For this review, take the finished solid that the model builds, in its own axes (mm). A direction names the side the tool comes from. Give positions to 0.01 mm unless a question says otherwise; leave off trailing zeros. Order: outer loops, then holes, each group sorted by start corner. A loop starts at its lowest first (then second) coordinate and runs counter-clockwise, first axis right, second up. Notation, with made-up numbers: (-3, 74.25) - (34, 74.25) arc R21 ccw to (34, 113.25) - close; hole circle Ø8 at (-18.75, 22). An arc over 180 degrees is marked (long way). Answer as a JSON object with one key per item and string values. Group by question number.
from build123d import *

# Parameters (mm, degrees)
F0_R     = 6.35
F1_DEPTH = 2.54
F2_R     = 3.175
F3_DEPTH = 5.08
F4_R     = 3.175
F4_W     = 17.78
F4_H     = 12.7
F5_DEPTH = 5.08
F7_R     = 5.07999
F8_R     = 3.175
F9_DEPTH = 5.08


# Not quite as in the source:
# - a fillet or chamfer is up to 0.001 mm smaller than in the source, because OpenCascade refuses the exact size


with BuildPart() as f1:
    # F0 (on Front) → F1 (new body)
    with BuildSketch(Plane.XZ):
        with Locations((0, 22.225)):
            Circle(F0_R)
    extrude(amount=F1_DEPTH)

    # F2 (on face) → F3 (join)
    with BuildSketch(Plane.XZ.offset(2.54)):
        with Locations((0, 22.225)):
            Circle(F2_R)
    extrude(amount=F3_DEPTH)

    # F4 (on face) → F5 (join)
    with BuildSketch(Plane.XZ.offset(7.62)):
        with BuildLine():
            ThreePointArc((4.9490759915, 23.3708825552), (5.0471628682, 22.8016688665), (5.08, 22.225))
            ThreePointArc((5.08, 22.225), (-0.5766688665, 17.1778371318), (-4.9490759915, 23.3708825552))
            Line((-4.9490759915, 23.3708825552), (-8.89, 6.35))
            Line((-8.89, 6.35), (8.89, 6.35))
            Line((8.89, 6.35), (4.9490759915, 23.3708825552))
        make_face()
        with BuildLine():
            ThreePointArc((-4.9490759915, 23.3708825552), (-0.5766688665, 17.1778371318), (5.08, 22.225))
            ThreePointArc((5.08, 22.225), (5.0471628682, 22.8016688665), (4.9490759915, 23.3708825552))
            ThreePointArc((4.9490759915, 23.3708825552), (0, 27.305), (-4.9490759915, 23.3708825552))
        make_face()
        with Locations((0, 22.225)):
            Circle(F4_R, mode=Mode.SUBTRACT)
        with Locations((0, 22.225)):
            Circle(F4_R)
        Rectangle(F4_W, F4_H)
    extrude(amount=F5_DEPTH)

    # F6: F1 across plane


with BuildPart() as f1_1:
    add(f1.part)
    add(f1.part.mirror(Plane.XY))

    # F7 (radius 5.08 in the source; OpenCascade refuses exactly that, so slightly less here)
    f7_edges = [f1_1.edges().sort_by_distance(p)[0] for p in [
        (-8.89, -12.7, 0),
        (8.89, -12.7, 0),
    ]]
    fillet(f7_edges, radius=F7_R)

    # F8 (on face) → F9 (join)
    with BuildSketch(Plane.XZ.offset(12.7)):
        Circle(F8_R)
    extrude(amount=F9_DEPTH)


solid = f1_1.part
1) Consider section B-B (x = 0). Give the boundary of the cut face in (y, z) (3 decimals), plus the area to 3 significant figures.
2) Consider section C-C (x = 5.5). Give the boundary of the cut face in (y, z).
3) For pin 1 (3 mm diameter, centred on y = -11.5, z = -0.5, fed in from -X); pin 2 (5 mm diameter, centred on x = 2.5, y = -6.5, fed in from +Z); pin 3 (10 mm diameter, centred on x = 1, z = 21, fed in from -Y), all flat-tipped, find the tip position at first contact; note any pin that passes through.
4) For line 1 (Y direction, x = -3, z = -21); line 2 (Y direction, x = -5, z = 20); line 3 (Y direction, x = 2.5, z = 8.5), list the stretches that pass through material, from the lowest coordinate up.
5) Mouldability with a two-part tool opening along Y and no side actions: class faces 1 (the face through (6.51, -9.51, -16.63)), 2 (the face through (0, -17.78, 0)), 3 (the face through (-3, -2.54, 24)) as released by +Y, released by -Y, zero draft, split by the parting line, or undercut.
6) Consider section A-A (z = -18). Give the boundary of the cut face in (x, y).
7) For faces 4 (the face through (-6.454, -9.511, -16.871)), 5 (the face through (0.096, -10.124, -27.304)), 6 (the face through (-1.377, -1.252, -16.026)), 7 (the face through (-2, -2.54, -25)), 8 (the face through (0.096, -10.124, 27.304)), list the 3-axis set-ups (+Z, -Z, +X, -X, +Y, -Y) from which the entire face can be reached by the end or side of a thin tool; tool diameter is ignored.
Result set:
{
 "1": {"outline": "(-17.78, -3.175) - (-12.7, -3.175) - (-12.7, -27.305) - (-7.62, -27.305) - (-7.62, -25.4) - (-2.54, -25.4) - (-2.54, -28.575) - (0, -28.575) - (0, -15.875) - (-2.54, -15.875) - (-2.54, -19.05) - (-7.62, -19.05) - (-7.62, 19.05) - (-2.54, 19.05) - (-2.54, 15.875) - (0, 15.875) - (0, 28.575) - (-2.54, 28.575) - (-2.54, 25.4) - (-7.62, 25.4) - (-7.62, 27.305) - (-12.7, 27.305) - (-12.7, 3.175) - (-17.78, 3.175) - close", "area": "439 mm2"},
 "2": {"outline": "(-12.41, -20.99) - (-7.62, -20.99) - (-7.62, 20.99) - (-12.41, 20.99) - close; (-2.54, -25.4) - (0, -25.4) - (0, -19.05) - (-2.54, -19.05) - close; (-2.54, 19.05) - (0, 19.05) - (0, 25.4) - (-2.54, 25.4) - close"},
 "3": {"pin 1": "stops at x = -8.3", "pin 2": "stops at z = 27.3", "pin 3": "stops at y = -12.7"},
 "4": {"line 1": "y = -12.7 to -7.62, -2.54 to 0", "line 2": "y = -12.56 to -7.62, -2.54 to 0", "line 3": "y = -12.7 to -7.62"},
 "5": {"face 1": "zero draft", "face 2": "released by -Y", "face 3": "undercut"},
 "6": {"outline": "(-6.19, -12.11) arc R5.08 ccw to (-3.81, -12.7) - (3.81, -12.7) arc R5.08 ccw to (6.19, -12.11) - (6.19, -7.62) - (-6.19, -7.62) - close; (-4.74, -2.54) - (4.74, -2.54) - (4.74, 0) - (-4.74, 0) - close"},
 "7": {"face 4": "-Z, -X, -Y", "face 5": "-Z, -Y", "face 6": "+Y", "face 7": "none", "face 8": "+Z, -Y"}
}
